Check sheet for the modelled part. Datum: model origin and axes. Units: mm. Face numbers are marked on the shaded views. Coordinates: 2 decimals unless noted, no trailing zeros. Order: outer loops, then holes, each group sorted by start corner. A loop starts at its lowest first (then second) coordinate and runs counter-clockwise, first axis right, second up.
1. Thickness scan on line 1 (X direction, y = -1, z = 0); line 2 (Z direction, x = 3, y = 4); line 3 (Z direction, x = 76.5, y = -1.5). Record the ranges inside material, lowest first.
2. Cross-section at B-B (z = 0). Enter the section's corners in (x, y).
3. Draft check along Z on the marked faces 1 and 2. Enter one of: released by +Z, released by -Z, zero draft, split by the parting line, or undercut.
4. Cross-section at C-C (y = 0). Enter the section's corners in (x, z), then the cut area to 3 significant figures.
5. Cross-section at A-A (x = 10). Enter the section's corners in (y, z).
6. Gauge pin test, flat ends, axial feed: pin 1 Ø5 at (x, y) = (66.5, -1.5) entering from -Z; pin 2 Ø1.5 at (x, y) = (47.5, 2) entering from +Z; pin 3 Ø8 at (x, z) = (0, 0) entering from +Y. Record the tip position at first contact, or that the pin passes through.
7. Cross-section at D-D (x = 25). Enter the section's corners in (y, z).
```python
from build123d import *

# Parameters (mm, degrees)
SKETCH2_R                = 2.5
SKETCH3_R                = 2.5
BOSS_EXTRUDE1_DEPTH      = 5
BOSS_EXTRUDE1_DEPTH_BACK = 5
SKETCH4_R                = 12.5
SKETCH5_R                = 5
CUT_EXTRUDE1_DEPTH       = 160.393381385


with BuildPart() as part:
    # Sweep1: sweep along a path in Sketch1
    with BuildLine(Plane(origin=(0, 0, 0), x_dir=(1, 0, 0), z_dir=(0, 1, 0))) as sweep1_path:
        Line((0, 0), (0, -90))
        Line((0, -90), (0, -130))
        ThreePointArc((0, -130), (1.464466094, -133.535533906), (5, -135))
        Line((5, -135), (80, -135))
    # Sketch2 → Sweep1 (sweep)
    with BuildSketch(Plane(origin=(80, 0, 135), x_dir=(0, 0, -1), z_dir=(1, 0, 0))):
        Circle(SKETCH2_R)
    sweep(path=sweep1_path.line)

    # Sweep2: sweep along a path in Sketch1_4
    with BuildLine(Plane(origin=(0, 0, 0), x_dir=(1, 0, 0), z_dir=(0, 1, 0))) as sweep2_path:
        Line((0, -90), (80, -90))
    # Sketch3 → Sweep2 (sweep)
    with BuildSketch(Plane(origin=(80, 0, 135), x_dir=(0, 0, -1), z_dir=(1, 0, 0))):
        with Locations((45, 0)):
            Circle(SKETCH3_R)
    sweep(path=sweep2_path.line)

    # Sketch4 → Boss-Extrude1 (add, two sides: drawn at the far end of the back side and taken through both)
    with BuildSketch(Plane(origin=(0, 0, 0), x_dir=(1, 0, 0), z_dir=(0, 1, 0)).offset(-BOSS_EXTRUDE1_DEPTH_BACK)):
        with Locations(Location((0, 0, 0), (0, 0, 270))):
            Circle(SKETCH4_R)
    extrude(amount=BOSS_EXTRUDE1_DEPTH + BOSS_EXTRUDE1_DEPTH_BACK)

    # Sketch5 → Cut-Extrude1 (cut, through all)
    with BuildSketch(Plane(origin=(0, 5, 0), x_dir=(1, 0, 0), z_dir=(0, 1, 0))):
        with Locations(Location((0, 0, 0), (0, 0, 270))):
            Circle(SKETCH5_R)
    extrude(amount=-CUT_EXTRUDE1_DEPTH, mode=Mode.SUBTRACT)


solid = part.part
```
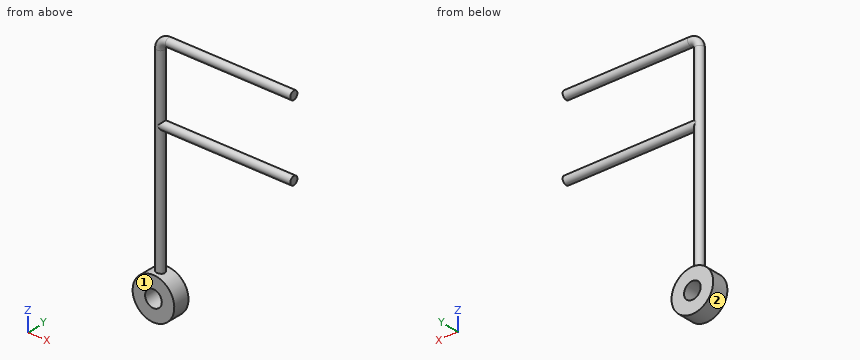
Data:
1. line 1: x = -12.5 to -5, 5 to 12.5
1. line 2: z = -12.13 to -4, 4 to 12.13
1. line 3: z = 88 to 92, 133 to 137
2. outline: (-12.5, -5) - (-5, -5) - (-5, 5) - (-12.5, 5) - close; (5, -5) - (12.5, -5) - (12.5, 5) - (5, 5) - close
3. face 1: zero draft
3. face 2: undercut
4. outline: (-2.5, 12.25) arc R12.5 ccw (long way) to (2.5, 12.25) - (2.5, 87.5) - (80, 87.5) - (80, 92.5) - (2.5, 92.5) - (2.5, 130) arc R2.5 cw to (5, 132.5) - (80, 132.5) - (80, 137.5) - (5, 137.5) arc R7.5 ccw to (-2.5, 130) - close; hole circle Ø10 at (0, 0)
4. area: 1,800 mm2
5. outline: (-5, -7.5) - (5, -7.5) - (5, 7.5) - (-5, 7.5) - close; circle Ø5 at (0, 90); circle Ø5 at (0, 135)
6. pin 1: stops at z = 87.5
6. pin 2: stops at z = 137.17
6. pin 3: passes through
7. outline: circle Ø5 at (0, 90); circle Ø5 at (0, 135)
